Input: part model. Units: mm. Frame: model coordinates. A direction names the side the tool comes from. Coordinates: 2 decimals unless noted, no trailing zeros. Order: outer loops, then holes, each group sorted by start corner. A loop starts at its lowest first (then second) coordinate and runs counter-clockwise, first axis right, second up. Notation, with made-up numbers: M 27.25,49.25 L 57.25,49.25 A30 cw 57.25,78.25 Z; hole C 87,18 d7. An arc over 180 degrees is marked long. Answer in a Markdown table with one row per item.
from build123d import *

# Parameters (mm, degrees)
F1_DEPTH = 10


with BuildPart() as f1:
    # F0 (on Top) → F1 (new body)
    with BuildSketch(Plane.XY):
        with BuildLine():
            ThreePointArc((-12.5, -10.3), (-12.3325349715, -11.1419035512), (-11.8556349186, -11.8556349186))
            Line((-11.8556349186, -11.8556349186), (-10.9722718241, -10.9722718241))
            ThreePointArc((-10.9722718241, -10.9722718241), (-10.9722718241, -9.0277281759), (-9.0277281759, -9.0277281759))
            Line((-9.0277281759, -9.0277281759), (-8.4852813742, -8.4852813742))
            ThreePointArc((-8.4852813742, -8.4852813742), (-11.5911099155, -3.1058285412), (-11.5911099155, 3.1058285412))
            ThreePointArc((-11.5911099155, 3.1058285412), (-11.2020379419, 4.3028299931), (-10.6897288112, 5.4524946533))
            ThreePointArc((-10.6897288112, 5.4524946533), (-9.7066834051, 7.0555153797), (-8.4852813742, 8.4852813742))
            Line((-8.4852813742, 8.4852813742), (-9.0277281759, 9.0277281759))
            ThreePointArc((-9.0277281759, 9.0277281759), (-10.9722718241, 9.0277281759), (-10.9722718241, 10.9722718241))
            Line((-10.9722718241, 10.9722718241), (-11.8556349186, 11.8556349186))
            ThreePointArc((-11.8556349186, 11.8556349186), (-12.3325349715, 11.1419035512), (-12.5, 10.3))
            Line((-12.5, 10.3), (-12.5, -10.3))
        make_face()
        with BuildLine():
            Line((-10.3, -12.5), (10.3, -12.5))
            ThreePointArc((10.3, -12.5), (11.1419035512, -12.3325349715), (11.8556349186, -11.8556349186))
            Line((11.8556349186, -11.8556349186), (10.9722718241, -10.9722718241))
            ThreePointArc((10.9722718241, -10.9722718241), (9.0277281759, -10.9722718241), (9.0277281759, -9.0277281759))
            Line((9.0277281759, -9.0277281759), (8.4852813742, -8.4852813742))
            ThreePointArc((8.4852813742, -8.4852813742), (6, -10.3923048454), (3.1058285412, -11.5911099155))
            ThreePointArc((3.1058285412, -11.5911099155), (1.8746588888, -11.8526644283), (0.6228655218, -11.9838240367))
            ThreePointArc((0.6228655218, -11.9838240367), (-4.3028299931, -11.2020379419), (-8.4852813742, -8.4852813742))
            Line((-8.4852813742, -8.4852813742), (-9.0277281759, -9.0277281759))
            ThreePointArc((-9.0277281759, -9.0277281759), (-8.7296656428, -9.4738102805), (-8.625, -10))
            ThreePointArc((-8.625, -10), (-9.4738102805, -11.2703343572), (-10.9722718241, -10.9722718241))
            Line((-10.9722718241, -10.9722718241), (-11.8556349186, -11.8556349186))
            ThreePointArc((-11.8556349186, -11.8556349186), (-11.1419035512, -12.3325349715), (-10.3, -12.5))
        make_face()
        with BuildLine():
            Line((10.9722718241, -10.9722718241), (11.8556349186, -11.8556349186))
            ThreePointArc((11.8556349186, -11.8556349186), (12.3325349715, -11.1419035512), (12.5, -10.3))
            Line((12.5, -10.3), (12.5, 10.3))
            ThreePointArc((12.5, 10.3), (12.3325349715, 11.1419035512), (11.8556349186, 11.8556349186))
            Line((11.8556349186, 11.8556349186), (10.9722718241, 10.9722718241))
            ThreePointArc((10.9722718241, 10.9722718241), (11.2703343572, 10.5261897195), (11.375, 10))
            ThreePointArc((11.375, 10), (10.5261897195, 8.7296656428), (9.0277281759, 9.0277281759))
            Line((9.0277281759, 9.0277281759), (8.4852813742, 8.4852813742))
            ThreePointArc((8.4852813742, 8.4852813742), (9.3273790531, 7.5498344353), (10.0668632893, 6.5313293834))
            ThreePointArc((10.0668632893, 6.5313293834), (11.5065711546, 3.4057040776), (12, 0))
            ThreePointArc((12, 0), (11.0865543901, -4.5922011884), (8.4852813742, -8.4852813742))
            Line((8.4852813742, -8.4852813742), (9.0277281759, -9.0277281759))
            ThreePointArc((9.0277281759, -9.0277281759), (10.5261897195, -8.7296656428), (11.375, -10))
            ThreePointArc((11.375, -10), (11.2703343572, -10.5261897195), (10.9722718241, -10.9722718241))
        make_face()
        with BuildLine():
            Line((10.9722718241, 10.9722718241), (11.8556349186, 11.8556349186))
            ThreePointArc((11.8556349186, 11.8556349186), (11.1419035512, 12.3325349715), (10.3, 12.5))
            Line((10.3, 12.5), (-10.3, 12.5))
            ThreePointArc((-10.3, 12.5), (-11.1419035512, 12.3325349715), (-11.8556349186, 11.8556349186))
            Line((-11.8556349186, 11.8556349186), (-10.9722718241, 10.9722718241))
            ThreePointArc((-10.9722718241, 10.9722718241), (-9.4738102805, 11.2703343572), (-8.625, 10))
            ThreePointArc((-8.625, 10), (-8.7296656428, 9.4738102805), (-9.0277281759, 9.0277281759))
            Line((-9.0277281759, 9.0277281759), (-8.4852813742, 8.4852813742))
            ThreePointArc((-8.4852813742, 8.4852813742), (0, 12), (8.4852813742, 8.4852813742))
            Line((8.4852813742, 8.4852813742), (9.0277281759, 9.0277281759))
            ThreePointArc((9.0277281759, 9.0277281759), (9.0277281759, 10.9722718241), (10.9722718241, 10.9722718241))
        make_face()
        with BuildLine():
            ThreePointArc((-10.6897288112, 5.4524946533), (-11.2020379419, 4.3028299931), (-11.5911099155, 3.1058285412))
            Line((-11.5911099155, 3.1058285412), (-5.7955549577, 1.5529142706))
            ThreePointArc((-5.7955549577, 1.5529142706), (-5.3311192747, 2.7530287465), (-4.6214557688, 3.8265057921))
            Line((-4.6214557688, 3.8265057921), (-10.6897288112, 5.4524946533))
        make_face()
        with BuildLine():
            Line((-5.7955549577, 1.5529142706), (0, 0))
            Line((0, 0), (-4.2426406871, 4.2426406871))
            ThreePointArc((-4.2426406871, 4.2426406871), (-4.4369295191, 4.0390167668), (-4.6214557688, 3.8265057921))
            ThreePointArc((-4.6214557688, 3.8265057921), (-5.3311192747, 2.7530287465), (-5.7955549577, 1.5529142706))
        make_face()
        with BuildLine():
            Line((-4.2426406871, 4.2426406871), (0, 0))
            Line((0, 0), (4.2426406871, 4.2426406871))
            ThreePointArc((4.2426406871, 4.2426406871), (0, 6), (-4.2426406871, 4.2426406871))
        make_face()
        with BuildLine():
            Line((0, 0), (4.2426406871, -4.2426406871))
            ThreePointArc((4.2426406871, -4.2426406871), (5.5432771951, -2.2961005942), (6, 0))
            ThreePointArc((6, 0), (5.9053989979, 1.0612552359), (5.6245791081, 2.0890452022))
            ThreePointArc((5.6245791081, 2.0890452022), (5.0497524692, 3.2403703492), (4.2426406871, 4.2426406871))
            Line((4.2426406871, 4.2426406871), (0, 0))
        make_face()
        with BuildLine():
            Line((5.6245791081, 2.0890452022), (10.0668632893, 6.5313293834))
            ThreePointArc((10.0668632893, 6.5313293834), (9.3273790531, 7.5498344353), (8.4852813742, 8.4852813742))
            Line((8.4852813742, 8.4852813742), (4.2426406871, 4.2426406871))
            ThreePointArc((4.2426406871, 4.2426406871), (5.0497524692, 3.2403703492), (5.6245791081, 2.0890452022))
        make_face()
        with BuildLine():
            ThreePointArc((1.5529142706, -5.7955549577), (3, -5.1961524227), (4.2426406871, -4.2426406871))
            Line((4.2426406871, -4.2426406871), (0, 0))
            Line((0, 0), (1.5529142706, -5.7955549577))
        make_face()
        with BuildLine():
            Line((0, 0), (-4.2426406871, -4.2426406871))
            ThreePointArc((-4.2426406871, -4.2426406871), (-2.7530287465, -5.3311192747), (-1.0031233393, -5.9155509943))
            ThreePointArc((-1.0031233393, -5.9155509943), (0.2813668055, -5.9933990957), (1.5529142706, -5.7955549577))
            Line((1.5529142706, -5.7955549577), (0, 0))
        make_face()
        with BuildLine():
            ThreePointArc((-5.7955549577, 1.5529142706), (-5.7955549577, -1.5529142706), (-4.2426406871, -4.2426406871))
            Line((-4.2426406871, -4.2426406871), (0, 0))
            Line((0, 0), (-5.7955549577, 1.5529142706))
        make_face()
        with BuildLine():
            ThreePointArc((0.6228655218, -11.9838240367), (1.8746588888, -11.8526644283), (3.1058285412, -11.5911099155))
            Line((3.1058285412, -11.5911099155), (1.5529142706, -5.7955549577))
            ThreePointArc((1.5529142706, -5.7955549577), (0.2813668055, -5.9933990957), (-1.0031233393, -5.9155509943))
            Line((-1.0031233393, -5.9155509943), (0.6228655218, -11.9838240367))
        make_face()
    extrude(amount=F1_DEPTH)


solid = f1.part
1) Mould query, pull axis X, two halves, no side actions, for faces 3 (the face through (-8.73, 2.34, 4.93)), 4 (the face through (12.5, 0, 5)), 5 (the face through (0, -12.5, 5)). Classes: +X half, -X half, draft (parallel to the pull), parting line (faces both ways), or undercut.
Resolved:
| item | result |
|---|---|
| face 3 | undercut |
| face 4 | +X half |
| face 5 | draft |
2) Material intervals for probe 1 along Y at (x, z) = (-10.25, 8.25); probe 2 along X at (y, z) = (-3.5, 7.25); probe 3 along Y at (x, z) = (-8, 4), sorted ascending.
Resolved:
| item | result |
|---|---|
| probe 1 | y = -12.5 to -11.35, -8.65 to -6.24, 2.75 to 5.33, 6.24 to 8.65, 11.35 to 12.5 |
| probe 2 | x = -12.5 to -11.48, -4.87 to 4.87, 11.48 to 12.5 |
| probe 3 | y = -12.5 to -8.94, 2.14 to 4.73, 8.94 to 12.5 |
3) Cut plane A-A, the plane x = -10. Output: boundary loops of the cut face in (y, z) (1 decimal), and give its area (3 significant figures).
Resolved:
| item | result |
|---|---|
| outline | M -12.5,0 L -11.4,0 L -11.4,10 L -12.5,10 Z; M -8.6,0 L -6.6,0 L -6.6,10 L -8.6,10 Z; M 2.7,0 L 5.3,0 L 5.3,10 L 2.7,10 Z; M 6.6,0 L 8.6,0 L 8.6,10 L 6.6,10 Z; M 11.4,0 L 12.5,0 L 12.5,10 L 11.4,10 Z |
| area | 88.2 mm2 |
4) Cut plane C-C, the plane z = 8. State how many separate pieces and enclosed holes the cut face has, and give its area (3 significant figures).
Resolved:
| item | result |
|---|---|
| separate pieces | 1 |
| enclosed holes | 7 |
| area | 303 mm2 |
5) Reachability of faces 1 (the face through (0, 12.5, 5)), 2 (the face through (6, 6, 5)) from +Z, -Z, +X, -X, +Y, -Y: full face, straight path, thin tool, end or side. Return the list, or none.
Resolved:
| item | result |
|---|---|
| face 1 | +Z, -Z, +X, -X, +Y |
| face 2 | +Z, -Z |
6) Cut plane B-B, the plane y = 8. Output: boundary loops of the cut face in (x, z).
Resolved:
| item | result |
|---|---|
| outline | M -12.5,0 L -8.94,0 L -8.94,10 L -12.5,10 Z; M 8,0 L 12.5,0 L 12.5,10 L 8,10 Z |
